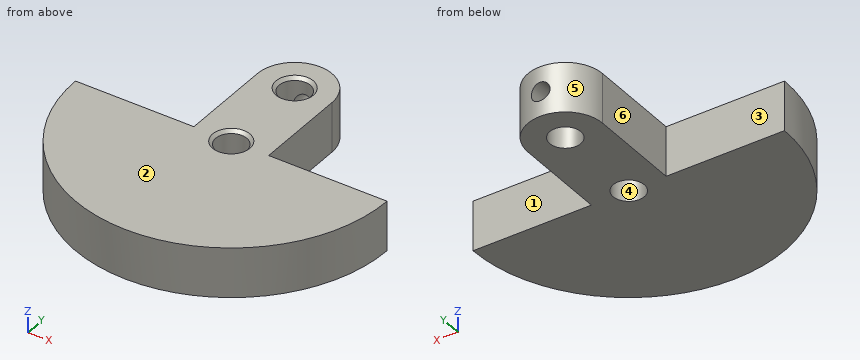
from build123d import *

# Parameters (mm, degrees)
SKETCH1_R           = 2.5
BOSS_EXTRUDE1_DEPTH = 8
CHAMFER1_SIZE       = 0.5
SKETCH2_R           = 1.5
CUT_EXTRUDE1_DEPTH  = 5


with BuildPart() as part:
    # Sketch1 → Boss-Extrude1 (new body)
    with BuildSketch(Plane.XY):
        with BuildLine():
            Line((-6, 15), (-6, 0))
            Line((-6, 0), (-25, 0))
            ThreePointArc((-25, 0), (0, -25), (25, 0))
            Line((25, 0), (6, 0))
            Line((6, 0), (6, 15))
            ThreePointArc((6, 15), (0, 21), (-6, 15))
        make_face()
        with Locations((0, 15)):
            Circle(SKETCH1_R, mode=Mode.SUBTRACT)
        Circle(SKETCH1_R, mode=Mode.SUBTRACT)
    extrude(amount=BOSS_EXTRUDE1_DEPTH)

    # Chamfer1
    chamfer1_edges = [part.edges().sort_by_distance(p)[0] for p in [
        (-2.5, 15, 8),
        (-2.5, 0, 8),
    ]]
    chamfer(chamfer1_edges, length=CHAMFER1_SIZE)

    # Sketch2 → Cut-Extrude1 (cut)
    with BuildSketch(Plane(origin=(0, 21, 0), x_dir=(1, 0, 0), z_dir=(0, 1, 0))):
        with Locations(Location((0, -4, 0), (0, 0, 270))):
            Circle(SKETCH2_R)
    extrude(amount=-CUT_EXTRUDE1_DEPTH, mode=Mode.SUBTRACT)


solid = part.part
Work out the finished part from the listing and answer in its coordinate system (mm). Face numbers are marked on the shaded views. A direction names the side the tool comes from. Round coordinates to 2 decimals unless told otherwise and drop trailing zeros. Loops run counter-clockwise (first coordinate to the right, second up) from the corner with the lowest first, then second, coordinate; pieces in that order, holes last. Notation, with made-up numbers: (72.25, 4) - (121.25, 4) arc R33 cw to (121.25, 43) - close; hole circle Ø8 at (-19, 10.5). An arc over 180 degrees is marked (long way). One line per item, written item: value.
Q1. The mould has two halves that part along Y. Classify the marked faces 4, 5 and 6: +Y half, -Y half, draft (parallel to the pull), parting line (faces both ways), or undercut.
Check values:
face 4: undercut
face 5: +Y half
face 6: draft
Q2. For the marked faces 1, 2 and 3, determine the directions among +Z, -Z, +X, -X, +Y, -Y from which every point of the face is accessible in a straight line to the end or side of a thin tool.
Check values:
face 1: +Z, -Z, +X, +Y
face 2: +Z, +X, -X, +Y, -Y
face 3: +Z, -Z, -X, +Y
Q3. Find section C-C on z = 4. Give the vertices of the cut face in (x, y).
Check values:
outline: (-25, 0) arc R25 ccw to (25, 0) - (6, 0) - (6, 15) arc R6 ccw to (1.5, 20.81) - (1.5, 17) arc R2.5 cw (long way) to (-1.5, 17) - (-1.5, 20.81) arc R6 ccw to (-6, 15) - (-6, 0) - close; hole circle Ø5 at (0, 0)
Q4. Each of these flat-tipped pins is pushed along its axis until it touches: pin 1 Ø2.5 at (y, z) = (5.5, 4) entering from -X; pin 2 Ø2.5 at (x, z) = (11.5, 2.5) entering from +Y; pin 3 Ø1 at (x, z) = (-17.5, 5.5) entering from -Y; pin 4 Ø3 at (x, y) = (0, 15) entering from +Z. Where does it stop, or does it pass through?
Check values:
pin 1: x = -6
pin 2: y = 0
pin 3: y = -18.33
pin 4: through
Q5. Find section A-A on z = 1.5. Give the vertices of the cut face in (x, y).
Check values:
outline: (-25, 0) arc R25 ccw to (25, 0) - (6, 0) - (6, 15) arc R6 ccw to (-6, 15) - (-6, 0) - close; hole circle Ø5 at (0, 0); hole circle Ø5 at (0, 15)
Q6. Straight lines are drawn through the part: probe 1 along Y at (x, z) = (0, 2.25); probe 2 along Z at (x, y) = (0, 19.35); probe 3 along Y at (x, z) = (0, 4). For each, find the intervals that lie inside material, in ascending order.
Check values:
probe 1: -25 to -2.5, 2.5 to 12.5, 17.5 to 21
probe 2: 0 to 2.5, 5.5 to 8
probe 3: -25 to -2.5, 2.5 to 12.5
Q7. Find section D-D on y = 8. Give the vertices of the cut face in (x, z).
Check values:
outline: (-6, 0) - (6, 0) - (6, 8) - (-6, 8) - close
Q8. Find section B-B on x = 0. Give the vertices of the cut face in (y, z), and give its area (3 significant figures).
Check values:
outline: (-25, 0) - (-2.5, 0) - (-2.5, 7.5) - (-3, 8) - (-25, 8) - close; (2.5, 0) - (12.5, 0) - (12.5, 7.5) - (12, 8) - (3, 8) - (2.5, 7.5) - close; (17.5, 0) - (21, 0) - (21, 2.5) - (17.5, 2.5) - close; (17.5, 5.5) - (21, 5.5) - (21, 8) - (18, 8) - (17.5, 7.5) - close
area: 277 mm2
